Build history of the part. All positions in model axes, mm. Give positions to 0.01 mm unless a question says otherwise; leave off trailing zeros. Write each loop counter-clockwise with the first axis right and the second up, starting at its lowest first coordinate (ties: lowest second). Pieces come first, ordered by that corner, then holes. Notation, with made-up numbers: M 11,57 L 41,57 A32 ccw 41,93 Z; hole C 32,43 d7. An arc over 180 degrees is marked long. Return JSON: item names as keys, results as strings. Group by question number.
Q1. Flat gauge pins, fed straight in: pin 1 Ø1 at (x, z) = (26, 707) entering from +Y; pin 2 Ø1.9 at (x, y) = (-51, -2.5) entering from -Z; pin 3 Ø1.5 at (y, z) = (-4.5, -14) entering from +X. Where does each tip first touch, or does it go through?
Q2. Band-saw the part on B-B, the plane z = 324. Give the cut face in (x, y), then the cut area to 3 significant figures.
Q3. Band-saw the part on A-A, the plane y = -2. Give the cut face in (x, z), then the cut area to 3 significant figures.
Q4. Wall check: probe 1 along X at (y, z) = (-3.25, 74.5); probe 2 along X at (y, z) = (-5.5, 120). Give the ranges that are in metal, low to high.
Q5. Band-saw the part on C-C, the plane x = -45. Give the cut face in (y, z).
from build123d import *

# Parameters (mm, degrees)
F1_DEPTH = 6.35


with BuildPart() as f1:
    # F0 (on Front) → F1 (new body)
    with BuildSketch(Plane.XZ):
        Polygon((0, -37.055038), (0, 877.344962), (-12.7, 877.344962), (-76.2, -37.055038), (-25.4, -37.055038), align=None)
        Polygon((12.7, 877.344962), (0, 877.344962), (0, -37.055038), (25.4, -37.055038), (76.2, -37.055038), align=None)
        Polygon((0, -113.255038), (0, -37.055038), (-25.4, -37.055038), (-12.7, -113.255038), align=None)
        Polygon((25.4, -37.055038), (0, -37.055038), (0, -113.255038), (12.7, -113.255038), align=None)
    extrude(amount=F1_DEPTH)


solid = f1.part
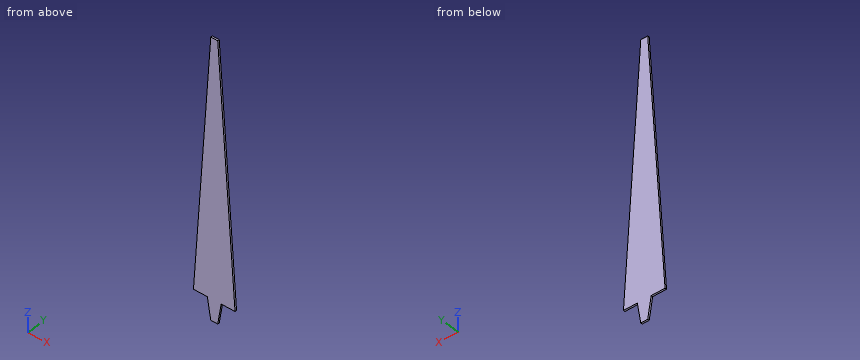
From the geometry:
{
 "1": {"pin 1": "passes through", "pin 2": "stops at z = -37.06", "pin 3": "stops at x = 74.65"},
 "2": {"outline": "M -51.13,-6.35 L 51.13,-6.35 L 51.13,0 L -51.13,0 Z", "area": "649 mm^2"},
 "3": {"outline": "M -76.2,-37.06 L -25.4,-37.06 L -12.7,-113.26 L 12.7,-113.26 L 25.4,-37.06 L 76.2,-37.06 L 12.7,877.34 L -12.7,877.34 Z", "area": "84,200 mm^2"},
 "4": {"probe 1": "x = -68.45 to 68.45", "probe 2": "x = -65.29 to 65.29"},
 "5": {"outline": "M -6.35,-37.06 L 0,-37.06 L 0,412.22 L -6.35,412.22 Z"}
}
